from build123d import *
from build123d.topology import SkipClean

# Parameters (mm, degrees)
SKETCH_1_W          = 65
SKETCH_1_H          = 53
SKETCH_1_R          = 1.6
EXTRUDE_1_DEPTH     = 4
EXTRUDE_2_DEPTH     = 60
SKETCH_5_R          = 1.6
SKETCH_5_R_2        = 11.5
CUT_EXTRUDE_1_DEPTH = 4
CUT_EXTRUDE_2_DEPTH = 69
SKETCH_6_3_R        = 1.6
EXTRUDE_3_DEPTH     = 4
EXTRUDE_START       = -53
EXTRUDE_4_DEPTH     = 4
SKETCH_7_R          = 2.1
CUT_EXTRUDE_3_DEPTH = 100
EXTRUDE_6_DEPTH     = 4
EXTRUDE_START_2     = -49
EXTRUDE_7_DEPTH     = 4
CUT_EXTRUDE_4_DEPTH = 70
FILLET_1_R          = 3


# Read off the part's stored shape, not the designer's step: 凸台-拉伸4
with BuildPart() as part:
    # 草图1 → 凸台-拉伸1 (new body)
    with BuildSketch(Plane.XY):
        Rectangle(SKETCH_1_W, SKETCH_1_H)
        with Locations((0, 13.5)):
            Circle(SKETCH_1_R, mode=Mode.SUBTRACT)
        with Locations((11.691342951, 6.75)):
            Circle(SKETCH_1_R, mode=Mode.SUBTRACT)
        with Locations((11.691342951, -6.75)):
            Circle(SKETCH_1_R, mode=Mode.SUBTRACT)
        with Locations((0, -13.5)):
            Circle(SKETCH_1_R, mode=Mode.SUBTRACT)
        with Locations((-11.691342951, -6.75)):
            Circle(SKETCH_1_R, mode=Mode.SUBTRACT)
        with Locations((-11.691342951, 6.75)):
            Circle(SKETCH_1_R, mode=Mode.SUBTRACT)
    extrude(amount=EXTRUDE_1_DEPTH)

    # 草图3 → 凸台-拉伸2 (add)
    with BuildSketch(Plane.XY.offset(4)):
        Polygon((28.5, 22.5), (-28.5, 22.5), (-32.5, 22.5), (-32.5, 26.5), (32.5, 26.5), (32.5, 22.5), align=None)
        Polygon((-28.5, -22.5), (28.5, -22.5), (32.5, -22.5), (32.5, -26.5), (-32.5, -26.5), (-32.5, -22.5), align=None)
    extrude(amount=EXTRUDE_2_DEPTH)

    # 草图5 → 切除-拉伸1 (cut)
    with BuildSketch(Plane.XZ.offset(26.5)):
        with Locations(Location((-17, 48, 0), (0, 0, 270))):
            Circle(SKETCH_5_R)
        with Locations(Location((-17, 30, 0), (0, 0, 270))):
            Circle(SKETCH_5_R_2)
        with Locations(Location((-4.272077939, 42.727922061, 0), (0, 0, 270))):
            Circle(SKETCH_5_R)
        with Locations(Location((1, 30, 0), (0, 0, 270))):
            Circle(SKETCH_5_R)
        with Locations(Location((-4.272077939, 17.272077939, 0), (0, 0, 270))):
            Circle(SKETCH_5_R)
        with Locations(Location((-17, 12, 0), (0, 0, 270))):
            Circle(SKETCH_5_R)
        with Locations(Location((-29.727922061, 17.272077939, 0), (0, 0, 270))):
            Circle(SKETCH_5_R)
        with Locations((-35, 30)):
            Circle(SKETCH_5_R)
        with Locations(Location((-29.727922061, 42.727922061, 0), (0, 0, 270))):
            Circle(SKETCH_5_R)
    extrude(amount=-CUT_EXTRUDE_1_DEPTH, mode=Mode.SUBTRACT)

    # 草图6 → 切除-拉伸2 (cut)
    with BuildSketch(Plane.XZ.offset(26.5)):
        with BuildLine():
            ThreePointArc((-32.5, 50.874625745), (-25.162711885, 54.685423527), (-17, 56))
            Line((-17, 56), (17, 56))
            ThreePointArc((17, 56), (25.162711885, 54.685423527), (32.5, 50.874625745))
            Line((32.5, 50.874625745), (32.5, 64))
            Line((32.5, 64), (-32.5, 64))
            Line((-32.5, 64), (-32.5, 50.874625745))
        make_face()
    extrude(amount=-CUT_EXTRUDE_2_DEPTH, mode=Mode.SUBTRACT)

    # 草图6<3> → 凸台-拉伸3 (add)
    # profile 1 of 2: a face of its own
    with BuildSketch(Plane.XZ.offset(26.5)):
        with BuildLine():
            Line((-32.5, 9.125374255), (-32.5, 50.874625745))
            ThreePointArc((-32.5, 50.874625745), (-43, 30), (-32.5, 9.125374255))
        make_face()
        with Locations(Location((-35, 30, 0), (0, 0, 270))):
            Circle(SKETCH_6_3_R, mode=Mode.SUBTRACT)
    # profile 2 of 2: a face of its own
    with BuildSketch(Plane.XZ.offset(26.5)):
        with BuildLine():
            ThreePointArc((32.5, 9.125374255), (43, 30), (32.5, 50.874625745))
            Line((32.5, 50.874625745), (32.5, 9.125374255))
        make_face()
    extrude(amount=-EXTRUDE_3_DEPTH)

    # 凸台-拉伸4 outline → 凸台-拉伸4 (add)
    with BuildSketch(Plane.XZ.offset(26.5).offset(EXTRUDE_START)):
        with BuildLine():
            Line((-32.5, 9.125374255), (-32.5, 50.874625745))
            ThreePointArc((-32.5, 50.874625745), (-43, 30), (-32.5, 9.125374255))
        make_face()
        with BuildLine():
            Line((32.5, 50.874625745), (32.5, 9.125374255))
            ThreePointArc((32.5, 9.125374255), (43, 30), (32.5, 50.874625745))
        make_face()
    extrude(amount=EXTRUDE_4_DEPTH)

    # 草图7 → 切除-拉伸3 (cut)
    with BuildSketch(Plane(origin=(0, 26.5, 0), x_dir=(1, 0, 0), z_dir=(0, 1, 0))):
        with Locations(Location((17, -30, 0), (0, 0, 270))):
            Circle(SKETCH_7_R)
    extrude(amount=-CUT_EXTRUDE_3_DEPTH, mode=Mode.SUBTRACT)

    # 草图8 → 凸台-拉伸6 (add)
    with BuildSketch(Plane.XZ.offset(26.5)):
        with BuildLine():
            ThreePointArc((4, 56), (0, 60), (-4, 56))
            Line((-4, 56), (-1.6, 56))
            ThreePointArc((-1.6, 56), (0, 57.6), (1.6, 56))
            Line((1.6, 56), (4, 56))
        make_face()
        with BuildLine():
            ThreePointArc((-42.950769231, 31.599242424), (-42.849150201, 32.796682655), (-42.692307692, 33.988148122))
            ThreePointArc((-42.692307692, 33.988148122), (-47, 30), (-42.692307692, 26.011851878))
            ThreePointArc((-42.692307692, 26.011851878), (-42.849150201, 27.203317345), (-42.950769231, 28.400757576))
            ThreePointArc((-42.950769231, 28.400757576), (-44.6, 30), (-42.950769231, 31.599242424))
        make_face()
        with BuildLine():
            ThreePointArc((42.692307692, 26.011851878), (47, 30), (42.692307692, 33.988148122))
            ThreePointArc((42.692307692, 33.988148122), (42.849150201, 32.796682655), (42.950769231, 31.599242424))
            ThreePointArc((42.950769231, 31.599242424), (44.113829154, 31.148644686), (44.6, 30))
            ThreePointArc((44.6, 30), (44.113829154, 28.851355314), (42.950769231, 28.400757576))
            ThreePointArc((42.950769231, 28.400757576), (42.849150201, 27.203317345), (42.692307692, 26.011851878))
        make_face()
    extrude(amount=-EXTRUDE_6_DEPTH)

    # 草图8<4> → 凸台-拉伸7 (add)
    with BuildSketch(Plane.XZ.offset(26.5).offset(EXTRUDE_START_2)):
        with BuildLine():
            ThreePointArc((4, 56), (0, 60), (-4, 56))
            Line((-4, 56), (-1.6, 56))
            ThreePointArc((-1.6, 56), (0, 57.6), (1.6, 56))
            Line((1.6, 56), (4, 56))
        make_face()
        with BuildLine():
            ThreePointArc((42.692307692, 26.011851878), (47, 30), (42.692307692, 33.988148122))
            ThreePointArc((42.692307692, 33.988148122), (42.849150201, 32.796682655), (42.950769231, 31.599242424))
            ThreePointArc((42.950769231, 31.599242424), (44.113829154, 31.148644686), (44.6, 30))
            ThreePointArc((44.6, 30), (44.113829154, 28.851355314), (42.950769231, 28.400757576))
            ThreePointArc((42.950769231, 28.400757576), (42.849150201, 27.203317345), (42.692307692, 26.011851878))
        make_face()
        with BuildLine():
            ThreePointArc((-42.950769231, 31.599242424), (-42.849150201, 32.796682655), (-42.692307692, 33.988148122))
            ThreePointArc((-42.692307692, 33.988148122), (-47, 30), (-42.692307692, 26.011851878))
            ThreePointArc((-42.692307692, 26.011851878), (-42.849150201, 27.203317345), (-42.950769231, 28.400757576))
            ThreePointArc((-42.950769231, 28.400757576), (-44.6, 30), (-42.950769231, 31.599242424))
        make_face()
    extrude(amount=-EXTRUDE_7_DEPTH)

    # 草图8<5> → 切除-拉伸4 (cut)
    with SkipClean():  # the faces are left unmerged after this step: merging them gives an invalid solid
        with BuildSketch(Plane.XZ.offset(26.5)):
            with BuildLine():
                Line((0, 56), (-1.6, 56))
                ThreePointArc((-1.6, 56), (-1.13137085, 54.86862915), (0, 54.4))
                Line((0, 54.4), (0, 56))
            make_face()
            with BuildLine():
                ThreePointArc((0, 54.4), (1.13137085, 54.86862915), (1.6, 56))
                Line((1.6, 56), (0, 56))
                Line((0, 56), (0, 54.4))
            make_face()
            with BuildLine():
                ThreePointArc((42.950769231, 28.400757576), (43, 30), (42.950769231, 31.599242424))
                ThreePointArc((42.950769231, 31.599242424), (41.4, 30), (42.950769231, 28.400757576))
            make_face()
            with BuildLine():
                ThreePointArc((44.6, 30), (44.113829154, 31.148644686), (42.950769231, 31.599242424))
                ThreePointArc((42.950769231, 31.599242424), (43, 30), (42.950769231, 28.400757576))
                ThreePointArc((42.950769231, 28.400757576), (44.113829154, 28.851355314), (44.6, 30))
            make_face()
            with BuildLine():
                ThreePointArc((-42.950769231, 28.400757576), (-43, 30), (-42.950769231, 31.599242424))
                ThreePointArc((-42.950769231, 31.599242424), (-44.6, 30), (-42.950769231, 28.400757576))
            make_face()
            with BuildLine():
                ThreePointArc((-41.4, 30), (-41.851355314, 31.113829154), (-42.950769231, 31.599242424))
                ThreePointArc((-42.950769231, 31.599242424), (-43, 30), (-42.950769231, 28.400757576))
                ThreePointArc((-42.950769231, 28.400757576), (-41.851355314, 28.886170846), (-41.4, 30))
            make_face()
        extrude(amount=-CUT_EXTRUDE_4_DEPTH, mode=Mode.SUBTRACT)

    # 圆角1
    fillet_1_edges = [part.edges().sort_by_distance(p)[0] for p in [
        (4, -24.5, 56),
        (-4, -24.5, 56),
        (-42.692307692, -24.5, 33.988148122),
        (-42.692307692, -24.5, 26.011851878),
        (42.692307692, -24.5, 26.011851878),
        (42.692307692, -24.5, 33.988148122),
        (-4, 24.5, 56),
        (4, 24.5, 56),
        (42.692307692, 24.5, 33.988148122),
        (42.692307692, 24.5, 26.011851878),
        (-42.692307692, 24.5, 26.011851878),
        (-42.692307692, 24.5, 33.988148122),
    ]]
    fillet(fillet_1_edges, radius=FILLET_1_R)


solid = part.part
Model file for the job. Use its own axes, mm. A direction names the side the tool comes from. Give positions to 0.01 mm unless a question says otherwise; leave off trailing zeros. Loops run counter-clockwise (first coordinate to the right, second up) from the corner with the lowest first, then second, coordinate; pieces in that order, holes last. Notation, with made-up numbers: (7, 23) -> (38, 23) arc R27 cw to (38, 56) -> close; hole circle Ø5 at (54.5, 66.25). An arc over 180 degrees is marked (long way). Use a Markdown table: item, result. Add a question column.
(1) Drop flat-ended pins along their axis: pin 1 Ø4 at (x, y) = (0, -13.5) entering from +Z; pin 2 Ø1.2 at (x, y) = (-11, -25) entering from +Z; pin 3 Ø3 at (x, z) = (-4.27, 42.73) entering from -Y. Give the stop position or say it passes through.
(2) Slice it at D-D on z = 52.5. List the corners of the cut face in (x, y), and give its area (3 significant figures).
(3) Tool access for faces 1 (the cylindrical face through (-4.9, -24.5, 15.8)), 2 (the flat face through (-1, 22.5, 32)), 3 (the flat face through (12, -25, 56)), 4 (the flat face through (-32.5, 0, 2)): list every direction of +Z, -Z, +X, -X, +Y, -Y with a clear straight run to the whole face (end or side of a thin tool).
(4) Slice it at C-C on y = 2.5. List the corners of the cut face in (x, z), and give its area (3 significant figures).
(5) Slice it at A-A on z = 6. List the corners of the cut face in (x, y), and give its area (3 significant figures).
(6) Slice it at B-B on x = -9. List the corners of the cut face in (y, z).
(7) Wall check: line 1 along Y through (x, z) = (0, 1.25); line 2 along Y through (x, z) = (23, 13.5); line 3 along Y through (x, z) = (-10, 39). Give the ranges that are in metal, low to high.
(8) Mould opens along X. For faces 5 (the cylindrical face through (-0.208, 15.086, 1.972)), 6 (the cylindrical face through (38.657, -24.528, 15.613)), 7 (the flat face through (0, 0, 0)) say: +X half, -X half, draft (parallel to the pull), parting line (faces both ways), or undercut.
Filled sheet:
| question | item | result |
|---|---|---|
| 1 | pin 1 | z = 4 |
| 1 | pin 2 | z = 56 |
| 1 | pin 3 | y = 22.5 |
| 2 | outline | (-30.03, -26.5) -> (30.03, -26.5) -> (30.03, -22.5) -> (-30.03, -22.5) -> close; (-30.03, 22.5) -> (30.03, 22.5) -> (30.03, 26.5) -> (-30.03, 26.5) -> close |
| 2 | area | 480 mm2 |
| 3 | face 1 | -Y |
| 3 | face 2 | +Z, +X, -X |
| 3 | face 3 | +Z, +X, +Y, -Y |
| 3 | face 4 | -Z, -X, +Y, -Y |
| 4 | outline | (-32.5, 0) -> (32.5, 0) -> (32.5, 4) -> (-32.5, 4) -> close |
| 4 | area | 260 mm2 |
| 5 | outline | (-32.5, -26.5) -> (32.5, -26.5) -> (32.5, -22.5) -> (-32.5, -22.5) -> close; (-32.5, 22.5) -> (32.5, 22.5) -> (32.5, 26.5) -> (-32.5, 26.5) -> close |
| 5 | area | 520 mm2 |
| 6 | outline | (-26.5, 0) -> (26.5, 0) -> (26.5, 56) -> (22.5, 56) -> (22.5, 4) -> (-22.5, 4) -> (-22.5, 21.74) -> (-26.5, 21.74) -> close; (-26.5, 38.26) -> (-22.5, 38.26) -> (-22.5, 56) -> (-26.5, 56) -> close |
| 7 | line 1 | -26.5 to -15.1, -11.9 to 11.9, 15.1 to 26.5 |
| 7 | line 2 | -26.5 to -22.5, 22.5 to 26.5 |
| 7 | line 3 | 22.5 to 26.5 |
| 8 | face 5 | undercut |
| 8 | face 6 | +X half |
| 8 | face 7 | draft |
